Here's the drawing with two shaded views (mm, measured from the low corner). I have some questions. A direction names the side the tool comes from. Round coordinates to 2 decimals unless told otherwise and drop trailing zeros. Order: outer loops, then holes, each group sorted by start corner. A loop starts at its lowest first (then second) coordinate and runs counter-clockwise, first axis right, second up. Notation, with made-up numbers: M 83.5,70 L 106.5,70 A35 cw 106.5,108 Z; hole C 22.25,31.5 d3. An arc over 180 degrees is marked long. One line per question, with ' | ' between items.
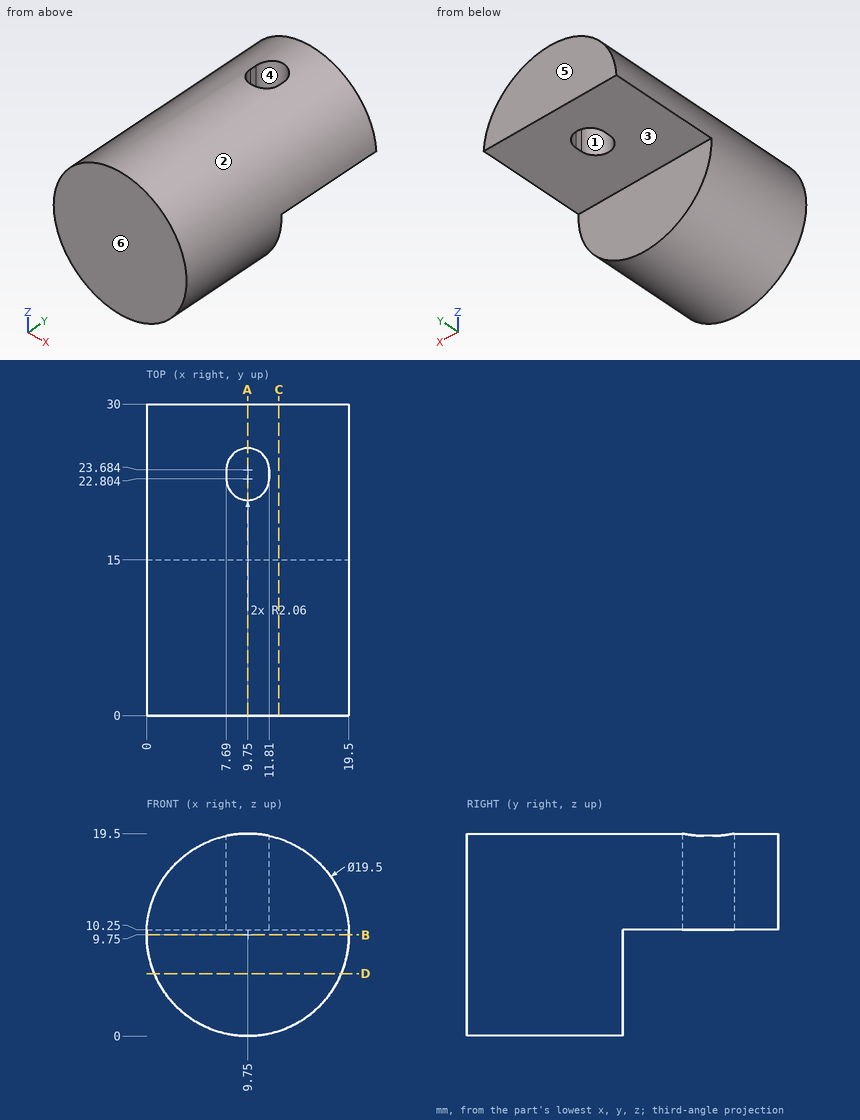
(1) If we section it at B-B on z = 9.75: Please give me the cut outline in (x, y), plus the area to 4 significant figures.
Final values:
outline: M 0,0 L 19.5,0 L 19.5,15 L 0,15 Z | area: 292.5 mm^2
(2) If we section it at A-A on x = 9.75: Please give me the cut outline in (y, z).
Final values:
outline: M 0,0 L 15,0 L 15,10.25 L 20.74,10.25 L 20.74,19.5 L 0,19.5 Z; M 25.74,10.25 L 30,10.25 L 30,19.5 L 25.74,19.5 Z
(3) Will these pins go through, and if not, where does the flat tip stop? pin 1 Ø1 at (y, z) = (6.5, 8) entering from -X; pin 2 Ø0.7 at (y, z) = (23.5, 15.5) entering from -X; pin 3 Ø2 at (x, z) = (16, 4) entering from +Y.
Final values:
pin 1: x = 0.08 | pin 2: x = 1.63 | pin 3: y = 15
(4) Thinking about a two-plate mould opening in Y: for the marked faces 4, 5 and 6, which applies, released by +Y, released by -Y, zero draft, split by the parting line, or undercut?
Final values:
face 4: undercut | face 5: released by +Y | face 6: released by -Y
(5) On a 3-axis mill with a long thin cutter (end or side, diameter ignored), from which of +Z, -Z, +X, -X, +Y, -Y can I reach the whole of each face in a straight line? I mean the marked faces 1, 2 and 3. Say none if no direction works.
Final values:
face 1: +Z, -Z | face 2: +Y, -Y | face 3: -Z, +X, -X, +Y
(6) If we section it at C-C on x = 12.75: Please give me the cut outline in (y, z), plus the area to 3 significant figures.
Final values:
outline: M 0,0.47 L 15,0.47 L 15,10.25 L 30,10.25 L 30,19.03 L 0,19.03 Z | area: 410 mm^2
(7) If we section it at D-D on z = 6: Please give me the cut outline in (x, y).
Final values:
outline: M 0.75,0 L 18.75,0 L 18.75,15 L 0.75,15 Z
(8) Please list where these lines run through material, in increasing order: probe 1 along Y at (x, z) = (12.5, 1.5); probe 2 along Z at (x, y) = (10, 11); probe 3 along Y at (x, z) = (8.5, 13.5). Write a range as [from, to].
Final values:
probe 1: [0, 15] | probe 2: [0, 19.5] | probe 3: [0, 21.17], [25.32, 30]
